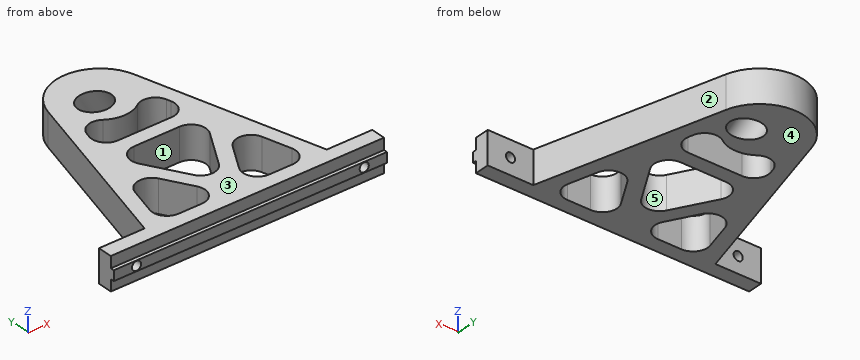
from build123d import *

# Parameters (mm, degrees)
F6_DEPTH       = 18
F7_W           = 150
F7_H           = 5.5
F7_R           = 2.5
F8_DEPTH       = 2
F9_DEPTH       = 8
F5_R           = 8
F10_DEPTH      = 40
F10_DEPTH_BACK = 30


with BuildPart() as f6:
    # F0 (on Top) → F6 (new body)
    with BuildSketch(Plane.XY):
        with BuildLine():
            Line((-75, -4), (75, -4))
            Line((75, -4), (75, 4))
            Line((75, 4), (50, 4))
            Line((50, 4), (23.6506350946, 102.3371685741))
            ThreePointArc((23.6506350946, 102.3371685741), (0, 120.484939165), (-23.6506350946, 102.3371685741))
            Line((-23.6506350946, 102.3371685741), (-50, 4))
            Line((-50, 4), (-75, 4))
            Line((-75, 4), (-75, -4))
        make_face()
        with BuildLine():
            ThreePointArc((-31.291987574, 4), (-37.6388142963, 7.1299085679), (-39.0193941843, 14.0705523608))
            Line((-39.0193941843, 14.0705523608), (-34.9566380514, 29.2329646678))
            ThreePointArc((-34.9566380514, 29.2329646678), (-28.2734409788, 35.0939711979), (-20.3010282108, 31.1624123069))
            Line((-20.3010282108, 31.1624123069), (-11.5470053838, 16))
            ThreePointArc((-11.5470053838, 16), (-11.5470053838, 8), (-18.4752086141, 4))
            Line((-18.4752086141, 4), (-31.291987574, 4))
        make_face(mode=Mode.SUBTRACT)
        with BuildLine():
            ThreePointArc((39.0193941843, 14.0705523608), (37.6388142963, 7.1299085679), (31.291987574, 4))
            Line((31.291987574, 4), (18.4752086141, 4))
            ThreePointArc((18.4752086141, 4), (11.5470053838, 8), (11.5470053838, 16))
            Line((11.5470053838, 16), (20.3010282108, 31.1624123069))
            ThreePointArc((20.3010282108, 31.1624123069), (28.2734409788, 35.0939711979), (34.9566380514, 29.2329646678))
            Line((34.9566380514, 29.2329646678), (39.0193941843, 14.0705523608))
        make_face(mode=Mode.SUBTRACT)
        with BuildLine():
            ThreePointArc((-19.4489291724, 45.6865334795), (-19.4489291724, 53.6865334795), (-12.5207259422, 57.6865334795))
            Line((-12.5207259422, 57.6865334795), (12.5207259422, 57.6865334795))
            ThreePointArc((12.5207259422, 57.6865334795), (19.4489291724, 53.6865334795), (19.4489291724, 45.6865334795))
            Line((19.4489291724, 45.6865334795), (6.9282032303, 24))
            ThreePointArc((6.9282032303, 24), (0, 20), (-6.9282032303, 24))
            Line((-6.9282032303, 24), (-19.4489291724, 45.6865334795))
        make_face(mode=Mode.SUBTRACT)
        with BuildLine():
            Line((14.7631307443, 65.6865334795), (-14.7631307443, 65.6865334795))
            ThreePointArc((-14.7631307443, 65.6865334795), (-21.1099574666, 68.8164420474), (-22.4905373546, 75.7570858403))
            Line((-22.4905373546, 75.7570858403), (-21.8677224991, 78.0814625246))
            ThreePointArc((-21.8677224991, 78.0814625246), (-16.8583855127, 83.5350112742), (-9.5202297882, 82.5419747342))
            ThreePointArc((-9.5202297882, 82.5419747342), (0, 79.515060835), (9.5202297882, 82.5419747342))
            ThreePointArc((9.5202297882, 82.5419747342), (16.8583855127, 83.5350112742), (21.8677224991, 78.0814625246))
            Line((21.8677224991, 78.0814625246), (22.4905373546, 75.7570858403))
            ThreePointArc((22.4905373546, 75.7570858403), (21.1099574666, 68.8164420474), (14.7631307443, 65.6865334795))
        make_face(mode=Mode.SUBTRACT)
    extrude(amount=F6_DEPTH)

    # F7 (on face) → F8 (join)
    with BuildSketch(Plane.XZ.offset(4)):
        with Locations((0, 9)):
            Rectangle(F7_W, F7_H)
        with Locations((-62.5, 9)):
            Circle(F7_R, mode=Mode.SUBTRACT)
        with Locations((62.5, 9)):
            Circle(F7_R, mode=Mode.SUBTRACT)
    extrude(amount=F8_DEPTH)

    # F9 (cut): faces of the model
    f9_faces = [f6.faces().sort_by_distance(p)[0] for p in [
        (62.5, -4, 9),
        (-62.5, -4, 9),
    ]]
    extrude(f9_faces, amount=-F9_DEPTH, mode=Mode.SUBTRACT)

    # F5 (on face) → F10 (cut, two sides)
    with BuildSketch(Plane(origin=(3.146304925, 0, -5.4495599862), x_dir=(0.8660254038, 0, 0.5), z_dir=(0.5, 0, -0.8660254038))) as f10_sk:
        with Locations((6.2546720728, -96)):
            Circle(F5_R)
    extrude(amount=-F10_DEPTH, mode=Mode.SUBTRACT)
    extrude(f10_sk.sketch, amount=F10_DEPTH_BACK, mode=Mode.SUBTRACT)


solid = f6.part
Could you check a few things on this model? Use its own coordinates, in mm. Face numbers are marked on the shaded views. A direction names the side the tool comes from. Give positions to 0.01 mm unless a question says otherwise; leave off trailing zeros. Order: outer loops, then holes, each group sorted by start corner. A loop starts at its lowest first (then second) coordinate and runs counter-clockwise, first axis right, second up. Notation, with made-up numbers: (59.5, 48.5) - (113.5, 48.5) arc R24 ccw to (113.5, 75.5) - close; hole circle Ø4 at (21.5, -8.75). An arc over 180 degrees is marked (long way). One line per question, with ' | ' between items. Start each with the question number.
Item 1: Thinking about a two-plate mould opening in Y: for the marked faces 1, 2 and 3, which applies, pulls with the +Y half, pulls with the -Y half, needs draft (parallel to the pull), parting line crosses it, or undercut?
Item 2: I'm going to push flat-ended pins straight in: pin 1 Ø5.5 at (x, z) = (63.5, 10.5) entering from +Y; pin 2 Ø1.6 at (x, y) = (-5, -5) entering from -Z; pin 3 Ø6.5 at (x, z) = (23, 8.5) entering from +Y. Where does each tip first touch, or does it pass through?
Item 3: I need wall thicknesses on probe 1 along Z at (x, y) = (-62.5, -0.75); probe 2 along X at (y, z) = (81, 17.25); probe 3 along Y at (x, z) = (11.5, 5.75). Which ranges of each line are inside material? Lowest first, please. Write a range as [from, to].
Item 4: I want a section at D-D on x = -47. Write out the boundary of the cut face in (y, z).
Item 5: I want a section at C-C on z = 9. Give the number of separate pieces and of enclosed holes in the cut face, then the cut area to 3 significant figures.
Item 6: I want a section at B-B on y = 99.5. Write out the boundary of the cut face in (x, z).
Item 7: For the marked faces 4 and 5, which set-ups out of +Z, -Z, +X, -X, +Y, -Y let a thin tool reach every point of the face, with its end or its side?
Item 8: I want a section at A-A on x = 62.5. Write out the boundary of the cut face in (y, z), then the cut area to 3 significant figures.
Verdict:
1) face 1: undercut | face 2: pulls with the +Y half | face 3: needs draft
2) pin 1: y = 4 | pin 2: z = 6.25 | pin 3: y = 110.47
3) probe 1: [0, 6.5], [11.5, 18] | probe 2: [-29.37, -20.39], [-6.84, 6.84], [20.39, 29.37] | probe 3: [-4, 8.08], [15.92, 31.92], [57.69, 65.69], [83.56, 91.45], [100.55, 117.62]
4) outline: (-6, 6.25) - (-4, 6.25) - (-4, 0) - (15.2, 0) - (15.2, 18) - (-4, 18) - (-4, 11.75) - (-6, 11.75) - close
5) separate pieces: 3 | enclosed holes: 5 | area: 5,940 mm^2
6) outline: (-24.41, 0) - (-1.08, 0) - (-11.48, 18) - (-24.41, 18) - close; (5.14, 18) - (15.53, 0) - (24.41, 0) - (24.41, 18) - close
7) face 4: -Z, +X, -X, +Y, -Y | face 5: +Z, -Z
8) outline: (-6, 6.25) - (-4, 6.25) - (-4, 0) - (4, 0) - (4, 6.5) - (-6, 6.5) - close; (-6, 11.5) - (4, 11.5) - (4, 18) - (-4, 18) - (-4, 11.75) - (-6, 11.75) - close | area: 105 mm^2
